Check sheet for the modelled part. Datum: model origin and axes. Units: mm. A direction names the side the tool comes from. Round coordinates to 2 decimals unless told otherwise and drop trailing zeros. Order: outer loops, then holes, each group sorted by start corner. A loop starts at its lowest first (then second) coordinate and runs counter-clockwise, first axis right, second up.
Q1. Depth check by flat-ended pin: P1, Ø4, axis at x = 30, z = 3, coming from the +Y side; P2, Ø2, axis at y = -2, z = 7, coming from the -X side; P3, Ø2.5, axis at x = 46.5, z = 3, coming from the -Y side; P4, Ø4, axis at x = 45.08, y = 0, coming from the +Z side. Enter the tip coordinate at first touch or a pass-through.
Q2. Cross-section at A-A on y = 0. Give the number of separate pieces and of enclosed holes in the cut face, then the cut area to 3 significant figures.
Q3. Mould release check, pull along X, two halves, no side actions. Record for faces 4 (the cylindrical face through (-11.6, -38.48, 2.46)), 5 (the cylindrical face through (46.32, 6.64, 7.1)), 6 (the cylindrical face through (-20.488, 47.634, 2.465)): +X half, -X half, draft (parallel to the pull), parting line (faces both ways), or undercut.
Q4. Set-up check for faces 1 (the flat face through (-29.68, 36.41, 2.46)), 2 (the cylindrical face through (-28.917, 36.796, 7.098)), 3 (the cylindrical face through (-11.45, 38.41, 2.46)): record each of +Z, -Z, +X, -X, +Y, -Y from which the full face is reachable in a straight line by a thin tool's end or side.
Q5. Scan lines: probe 1 along Y at (x, z) = (0, 4.25); probe 2 along Y at (x, z) = (-25.5, 4.25); probe 3 along X at (y, z) = (0.5, 6). Record each from-to range of solid material in increasing order.
Q6. Cross-section at B-B on z = 2.5. Record the cut outline in (x, y), then the cut area to 3 significant figures.
from build123d import *

# Parameters (mm, degrees)
SKETCH1_R           = 29.400000026
SKETCH1_R_2         = 3.5
BOSS_EXTRUDE1_DEPTH = 8
FILLET1_R           = 3


with BuildPart() as part:
    # Sketch1 → Boss-Extrude1 (new body)
    with BuildSketch(Plane.XY):
        with BuildLine():
            Line((-28.843288881, -34.9580418), (-30.495190528, -37.819219382))
            ThreePointArc((-30.495190528, -37.819219382), (-30.994692641, -41.613314607), (-28.665063509, -44.649346401))
            Line((-28.665063509, -44.649346401), (-24.334936491, -47.149346401))
            ThreePointArc((-24.334936491, -47.149346401), (-20.540841265, -47.648848513), (-17.504809472, -45.319219382))
            Line((-17.504809472, -45.319219382), (-15.852907825, -42.4580418))
            ThreePointArc((-15.852907825, -42.4580418), (-11.527824655, -38.446588336), (-5.694184248, -37.570949758))
            ThreePointArc((-5.694184248, -37.570949758), (19, -32.908965344), (35.384489059, -13.854166667))
            ThreePointArc((35.384489059, -13.854166667), (39.059634515, -9.239905166), (44.696196706, -7.5))
            Line((44.696196706, -7.5), (48, -7.5))
            ThreePointArc((48, -7.5), (51.535533906, -6.035533906), (53, -2.5))
            Line((53, -2.5), (53, 2.5))
            ThreePointArc((53, 2.5), (51.535533906, 6.035533906), (48, 7.5))
            Line((48, 7.5), (44.696196706, 7.5))
            ThreePointArc((44.696196706, 7.5), (39.059634515, 9.239905166), (35.384489059, 13.854166667))
            ThreePointArc((35.384489059, 13.854166667), (19, 32.908965344), (-5.694184248, 37.570949758))
            ThreePointArc((-5.694184248, 37.570949758), (-11.527824655, 38.446588336), (-15.852907825, 42.4580418))
            Line((-15.852907825, 42.4580418), (-17.504809472, 45.319219382))
            ThreePointArc((-17.504809472, 45.319219382), (-20.540841265, 47.648848513), (-24.334936491, 47.149346401))
            Line((-24.334936491, 47.149346401), (-28.665063509, 44.649346401))
            ThreePointArc((-28.665063509, 44.649346401), (-30.994692641, 41.613314607), (-30.495190528, 37.819219382))
            Line((-30.495190528, 37.819219382), (-28.843288881, 34.9580418))
            ThreePointArc((-28.843288881, 34.9580418), (-27.53180986, 29.20668317), (-29.690304811, 23.716783092))
            ThreePointArc((-29.690304811, 23.716783092), (-32.237173632, 20.118763287), (-34.35021834, 16.25))
            ThreePointArc((-34.35021834, 16.25), (-37.744312009, -4.400785266), (-29.690304811, -23.716783092))
            ThreePointArc((-29.690304811, -23.716783092), (-27.53180986, -29.20668317), (-28.843288881, -34.9580418))
        make_face()
        Circle(SKETCH1_R, mode=Mode.SUBTRACT)
        with Locations((45.084761958, 0)):
            Circle(SKETCH1_R_2, mode=Mode.SUBTRACT)
        with Locations((-22.542380979, -39.044549179)):
            Circle(SKETCH1_R_2, mode=Mode.SUBTRACT)
        with Locations((-22.542380979, 39.044549179)):
            Circle(SKETCH1_R_2, mode=Mode.SUBTRACT)
    extrude(amount=BOSS_EXTRUDE1_DEPTH)

    # Fillet1
    fillet1_edges = [part.edges().sort_by_distance(p)[0] for p in [
        (-27.53180986, 29.20668317, 8),
        (-27.53180986, -29.20668317, 8),
        (-29.669239705, -36.388630591, 8),
        (-30.994692641, -41.613314607, 8),
        (-26.5, -45.899346401, 8),
        (-20.540841265, -47.648848513, 8),
        (-16.678858648, -43.888630591, 8),
        (-11.527824655, -38.446588336, 8),
        (19, -32.908965344, 8),
        (39.059634515, -9.239905166, 8),
        (46.348098353, -7.5, 8),
        (-38, 0, 8),
        (51.535533906, -6.035533906, 8),
        (53, 0, 8),
        (51.535533906, 6.035533906, 8),
        (46.348098353, 7.5, 8),
        (39.059634515, 9.239905166, 8),
        (19, 32.908965344, 8),
        (-11.527824655, 38.446588336, 8),
        (-16.678858648, 43.888630591, 8),
        (-20.540841265, 47.648848513, 8),
        (-26.5, 45.899346401, 8),
        (-30.994692641, 41.613314607, 8),
        (-29.669239705, 36.388630591, 8),
    ]]
    fillet(fillet1_edges, radius=FILLET1_R)


solid = part.part
Results found:
1. P1: stops at y = 25.69
1. P2: stops at x = -37.78
1. P3: stops at y = -7.5
1. P4: passes through
2. separate pieces: 3
2. enclosed holes: 0
2. area: 198 mm2
3. face 4: undercut
3. face 5: draft
3. face 6: parting line
4. face 1: +Z, -Z, -X
4. face 2: +Z, -X
4. face 3: +Z, -Z, +Y
5. probe 1: y = -38 to -29.4, 29.4 to 38
5. probe 2: y = -46.48 to -40.92, -37.17 to -14.63, 14.63 to 37.17, 40.92 to 46.48
5. probe 3: x = -37.83 to -29.4, 29.4 to 41.62, 48.55 to 52.83
6. outline: (-30.5, -37.82) arc R5 ccw to (-28.67, -44.65) - (-24.33, -47.15) arc R5 ccw to (-17.5, -45.32) - (-15.85, -42.46) arc R10 cw to (-5.69, -37.57) arc R38 ccw to (35.38, -13.85) arc R10 cw to (44.7, -7.5) - (48, -7.5) arc R5 ccw to (53, -2.5) - (53, 2.5) arc R5 ccw to (48, 7.5) - (44.7, 7.5) arc R10 cw to (35.38, 13.85) arc R38 ccw to (-5.69, 37.57) arc R10 cw to (-15.85, 42.46) - (-17.5, 45.32) arc R5 ccw to (-24.33, 47.15) - (-28.67, 44.65) arc R5 ccw to (-30.5, 37.82) - (-28.84, 34.96) arc R10 cw to (-29.69, 23.72) arc R38 ccw to (-29.69, -23.72) arc R10 cw to (-28.84, -34.96) - close; hole circle Ø58.8 at (0, 0); hole circle Ø7 at (-22.54, -39.04); hole circle Ø7 at (-22.54, 39.04); hole circle Ø7 at (45.08, 0)
6. area: 2,420 mm2
